from build123d import *

# Parameters (mm, degrees)
F1_DEPTH = 762
F2_R     = 217.8858008063
F3_DEPTH = 508


# Not quite as in the source:
# - a feature names something its author has since deleted; it is built from what else it names


with BuildPart() as f1:
    # F0 (on Front) → F1 (new body)
    with BuildSketch(Plane.XZ):
        Polygon((-1270, 0), (0, 0), (0, 508), (-635, 508), (-635, 889), (-1270, 889), align=None)
    extrude(amount=F1_DEPTH)

    # F2 (on face) → F3 (cut)
    with BuildSketch(Plane.XY.offset(508)):
        with Locations((-295.0017750263, -381)):
            Circle(F2_R)
    extrude(amount=-F3_DEPTH, mode=Mode.SUBTRACT)


solid = f1.part
Geometry check sheet. Reference: the model listing, model coordinates, mm. A direction names the side the tool comes from. Give positions to 0.01 mm unless a question says otherwise; leave off trailing zeros. Write each loop counter-clockwise with the first axis right and the second up, starting at its lowest first coordinate (ties: lowest second). Pieces come first, ordered by that corner, then holes.
1) Cross-section at C-C (z = 198). Record the boundary of the cut face in (x, y), plus the area to 3 significant figures.
Values follow:
outline: (-1270, -762) - (0, -762) - (0, 0) - (-1270, 0) - close; hole circle Ø435.77 at (-295, -381)
area: 819,000 mm2
2) Cross-section at A-A (y = -381). Record the boundary of the cut face in (x, z).
Values follow:
outline: (-1270, 0) - (-512.89, 0) - (-512.89, 508) - (-635, 508) - (-635, 889) - (-1270, 889) - close; (-77.12, 0) - (0, 0) - (0, 508) - (-77.12, 508) - close
3) Set-up check for faces 5 (the face through (-525, -376, 508)), 6 (the face through (-785, -762, 352)): record each of +Z, -Z, +X, -X, +Y, -Y from which the full face is reachable in a straight line by a thin tool's end or side.
Values follow:
face 5: +Z, +X, +Y, -Y
face 6: +Z, -Z, +X, -X, -Y
4) Thickness scan on line 1 (X direction, y = -561, z = 798); line 2 (Z direction, x = -584, y = -439.5); line 3 (Y direction, x = -263, z = 253.5). Record the ranges inside material, lowest first.
Values follow:
line 1: x = -1270 to -635
line 2: z = 0 to 508
line 3: y = -762 to -596.52, -165.48 to 0
5) Go/stop test with a flat-tipped pin: pin 1 Ø8 at (x, y) = (-414, -560.5) entering from +Z. Record where the tip stops, or that it passes through.
Values follow:
pin 1: stops at z = 508
6) Release check for a two-part mould opening along X. For faces 1 (the face through (-455.59, -233.74, 257.56)), 2 (the face through (-1270, -376, 451)), 3 (the face through (0, -376, 250)), 4 (the face through (-644, -376, 0)) record: released by +X, released by -X, zero draft, split by the parting line, or undercut.
Values follow:
face 1: undercut
face 2: released by -X
face 3: released by +X
face 4: zero draft
7) Cross-section at B-B (x = -452). Record the boundary of the cut face in (y, z), plus the area to 3 significant figures.
Values follow:
outline: (-762, 0) - (-532.08, 0) - (-532.08, 508) - (-762, 508) - close; (-229.92, 0) - (0, 0) - (0, 508) - (-229.92, 508) - close
area: 234,000 mm2
8) Cross-section at D-D (y = -694.5). Record the boundary of the cut face in (x, z), plus the area to 3 significant figures.
Values follow:
outline: (-1270, 0) - (0, 0) - (0, 508) - (-635, 508) - (-635, 889) - (-1270, 889) - close
area: 887,000 mm2
